Here's how the part is built. I have some questions about the finished solid (model axes, mm). Face numbers are marked on the shaded views. A direction names the side the tool comes from. Round coordinates to 2 decimals unless told otherwise and drop trailing zeros. Order: outer loops, then holes, each group sorted by start corner. A loop starts at its lowest first (then second) coordinate and runs counter-clockwise, first axis right, second up. Notation, with made-up numbers: (25.5, 60.5) -> (81.5, 60.5) arc R23 cw to (81.5, 76.5) -> close; hole circle Ø5 at (57.25, 87). An arc over 180 degrees is marked (long way). Use a Markdown table: item, result. Add a question column.
(1) I want a section at C-C, the plane z = 1.25. Please give me the cut outline in (x, y), then the cut area to 3 significant figures.
(2) On a 3-axis mill with a long thin cutter (end or side, diameter ignored), from which of +Z, -Z, +X, -X, +Y, -Y can I reach the whole of each face in a straight line? I mean the marked faces 1, 2 and 3. Say none if no direction works.
(3) I want a section at B-B, the plane y = -0.75. Please give me the cut outline in (x, z), then the cut area to 3 significant figures.
(4) I want a section at D-D, the plane y = 2.25. Please give me the cut outline in (x, z).
(5) Thinking about a two-plate mould opening in Y: for the marked faces 4, 5, 6 and 7, which applies, pulls with the +Y half, pulls with the -Y half, needs draft (parallel to the pull), parting line crosses it, or undercut?
(6) If I drill on probe 1 along Y at (x, z) = (15, -2.25); probe 2 along X at (y, z) = (-1.5, -4.75); probe 3 along Z at (x, y) = (1.5, 3.25), over which ranges is the centre line in solid material (lowest first)?
(7) I'm going to push flat-ended pins straight in: P1, Ø1, axis at x = 11.5, y = -0.5, coming from the -Z side; P2, Ø2, axis at x = -1.5, y = 2.5, coming from the -Z side; P3, Ø1.1, axis at y = -1.5, z = -4, coming from the -X side. Where does each tip first touch, or does it pass through?
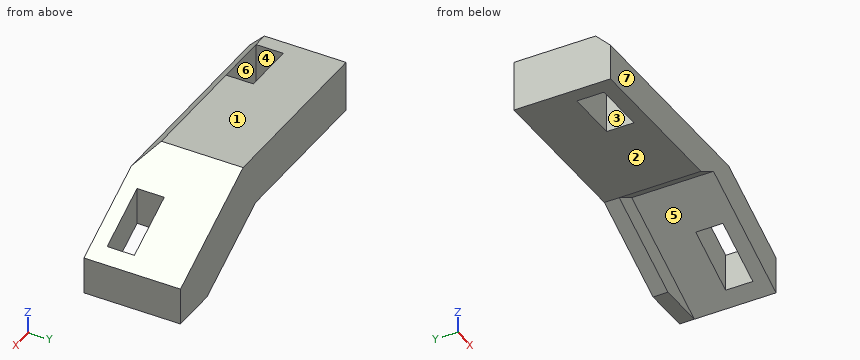
from build123d import *

# Parameters (mm, degrees)
SKETCH1_W               = 13
SKETCH1_H               = 4.1
BOSS_EXTRUDE1_DEPTH     = 3.9
CUT_EXTRUDE1_DEPTH      = 6.6
CUT_EXTRUDE2_DEPTH      = 20.434185635
CUT_EXTRUDE2_DEPTH_BACK = 20.434185635
SKETCH3_W               = 4.3
SKETCH3_H               = 2.2
CHAMFER1_SIZE           = 1.2


with BuildPart() as part:
    # Sketch1 → Boss-Extrude1 (new, symmetric)
    with BuildSketch(Plane(origin=(0, 0, 0), x_dir=(1, 0, 0), z_dir=(0, 1, 0))):
        Polygon((13.499620547, 5.899061033), (17.3, 5.899061033), (17.3, 2.899061033), (8.3, -2.05), (6.5, -2.05), (6.5, 2.05), align=None)
        Rectangle(SKETCH1_W, SKETCH1_H)
    extrude(amount=BOSS_EXTRUDE1_DEPTH, both=True)

    # Sketch2 → Cut-Extrude1 (cut)
    with BuildSketch(Plane.XZ.offset(3.9)):
        Polygon((17.3, -5.899061033), (8.3, -0.95), (6.5, -2.05), (13.499620547, -5.899061033), align=None)
    extrude(amount=-CUT_EXTRUDE1_DEPTH, mode=Mode.SUBTRACT)

    # Sketch3 → Cut-Extrude2 (cut, two sides: drawn at the far end of the back side and taken through both)
    with BuildSketch(Plane.XY.offset(2.05).offset(-CUT_EXTRUDE2_DEPTH_BACK)):
        with Locations((-3.15, -1.6)):
            Rectangle(SKETCH3_W, SKETCH3_H)
        with Locations((13.95, -1.6)):
            Rectangle(SKETCH3_W, SKETCH3_H)
    extrude(amount=CUT_EXTRUDE2_DEPTH + CUT_EXTRUDE2_DEPTH_BACK, mode=Mode.SUBTRACT)

    # Chamfer1
    chamfer1_edges = [part.edges().sort_by_distance(p)[0] for p in [
        (0.9, -3.9, 2.05),
    ]]
    chamfer(chamfer1_edges, length=CHAMFER1_SIZE - 0.0001)  # a hair under: the kernel refuses the full size


solid = part.part
Taken from the geometry:
| question | item | result |
|---|---|---|
| 1 | outline | (-6.5, -3.5) -> (9.75, -3.5) -> (9.75, 3.9) -> (-6.5, 3.9) -> close; hole (-5.3, -2.7) -> (-1, -2.7) -> (-1, -0.5) -> (-5.3, -0.5) -> close |
| 1 | area | 111 mm2 |
| 2 | face 1 | +Z, +X, -X, +Y, -Y |
| 2 | face 2 | -Z, -X, +Y, -Y |
| 2 | face 3 | +Z, -Z |
| 3 | outline | (-6.5, -2.05) -> (-5.3, -2.05) -> (-5.3, 2.05) -> (-6.5, 2.05) -> close; (-1, -2.05) -> (6.5, -2.05) -> (8.3, -0.95) -> (11.8, -2.87) -> (11.8, 0.13) -> (8.3, 2.05) -> (-1, 2.05) -> close; (16.1, -5.24) -> (17.3, -5.9) -> (17.3, -2.9) -> (16.1, -2.24) -> close |
| 3 | area | 56.2 mm2 |
| 4 | outline | (-6.5, -2.05) -> (6.5, -2.05) -> (8.3, -0.95) -> (17.3, -5.9) -> (17.3, -2.9) -> (8.3, 2.05) -> (-6.5, 2.05) -> close |
| 5 | face 4 | undercut |
| 5 | face 5 | needs draft |
| 5 | face 6 | undercut |
| 5 | face 7 | pulls with the -Y half |
| 6 | probe 1 | y = -3.9 to -2.7, -0.5 to 3.9 |
| 6 | probe 2 | x = 16.1 to 17.3 |
| 6 | probe 3 | z = -2.05 to 2.05 |
| 7 | P1 | stops at z = -2.98 |
| 7 | P2 | stops at z = -2.05 |
| 7 | P3 | stops at x = 16.1 |
